Read the model definition and answer for the solid it produces. Units are mm, in the model's axes. A direction names the side the tool comes from. Coordinates: 2 decimals unless noted, no trailing zeros. Order: outer loops, then holes, each group sorted by start corner. A loop starts at its lowest first (then second) coordinate and runs counter-clockwise, first axis right, second up. Notation, with made-up numbers: M 3,-22.75 L 30,-22.75 A22 ccw 30,14.25 Z; hole C 28.5,3.5 d2. An arc over 180 degrees is marked long. Put each result on its own line as item: value.
from build123d import *

# Parameters (mm, degrees)
CYLINDER001_R      = 10.5
CYLINDER001_DEPTH  = 25
CYLINDER_R         = 26
CYLINDER_DEPTH     = 25
CYLINDER002_R      = 30
CYLINDER002_DEPTH  = 5
SKETCH_R           = 6
POCKET_DEPTH       = 40
POLARPATTERN_COUNT = 8


with BuildPart() as cylinder001:
    # Cylinder001 → Cylinder001 (new body)
    with BuildSketch(Plane.XY):
        Circle(CYLINDER001_R)
    extrude(amount=CYLINDER001_DEPTH)


with BuildPart() as cylinder:
    # Cylinder → Cylinder (new body)
    with BuildSketch(Plane.XY):
        Circle(CYLINDER_R)
    extrude(amount=CYLINDER_DEPTH)


with BuildPart() as polarpattern:
    # Cylinder002 → Cylinder002 (new body)
    with BuildSketch(Plane.XY):
        Circle(CYLINDER002_R)
    extrude(amount=CYLINDER002_DEPTH)

    # Fusion: union Cylinder
    add(cylinder.part)

    # Cut: cut Cylinder001
    add(cylinder001.part, mode=Mode.SUBTRACT)

    # Sketch → Pocket (cut)
    with BuildSketch(Plane.XY.offset(25)):
        with Locations((0, 18.25)):
            Circle(SKETCH_R)
    pocket = extrude(amount=-POCKET_DEPTH, mode=Mode.SUBTRACT)

    # PolarPattern: Pocket ×8 about axis
    polarpattern_axis = Axis((0, 0, 25), (0, 0, 1))
    for i in range(1, POLARPATTERN_COUNT):
        add(pocket.rotate(polarpattern_axis, i * 360 / POLARPATTERN_COUNT), mode=Mode.SUBTRACT)


solid = polarpattern.part
Q1. Find section A-A on y = 0. Write down the section's boundary in (x, z), plus the area to 3 significant figures.
Answers below:
outline: M -30,0 L -24.25,0 L -24.25,25 L -26,25 L -26,5 L -30,5 Z; M -12.25,0 L -10.5,0 L -10.5,25 L -12.25,25 Z; M 10.5,0 L 12.25,0 L 12.25,25 L 10.5,25 Z; M 24.25,0 L 30,0 L 30,5 L 26,5 L 26,25 L 24.25,25 Z
area: 215 mm^2
Q2. A tool of negligible diameter and unlimited length cuts with its end or side. For faces 4 (the face through (-9, 25, 5)), 5 (the face through (-29.97, 1.32, 2.46)), from which of +Z, -Z, +X, -X, +Y, -Y can it reach the whole face along a straight path? Write none if from no direction.
Answers below:
face 4: +Z
face 5: +Z, -Z
Q3. Consider line 1 along Y through (x, z) = (0, 19.75); line 2 along Y through (x, z) = (2, 2.25); line 3 along Y through (x, z) = (-11.5, 2.5). Determine where each line is inside the solid, lowest interval first.
Answers below:
line 1: y = -26 to -24.25, -12.25 to -10.5, 10.5 to 12.25, 24.25 to 26
line 2: y = -29.93 to -23.91, -12.59 to -10.31, 10.31 to 12.59, 23.91 to 29.93
line 3: y = -27.71 to -18.74, -7.07 to 7.07, 18.74 to 27.71
Q4. Find section C-C on x = 22. Write down the section's boundary in (y, z), plus the area to 3 significant figures.
Answers below:
outline: M -20.4,0 L -4.68,0 L -4.68,25 L -13.86,25 L -13.86,5 L -20.4,5 Z; M 4.68,0 L 20.4,0 L 20.4,5 L 13.86,5 L 13.86,25 L 4.68,25 Z
area: 524 mm^2
Q5. Find section D-D on z = 3.5. Give the number of separate pieces and of enclosed holes in the cut face, plus the area to 3 significant figures.
Answers below:
separate pieces: 1
enclosed holes: 9
area: 1,580 mm^2
Q6. For a pull along X with two mould halves and no side action, classify faces 1 (the face through (-15.95, 5.54, 12.68)), 2 (the face through (11, 0, 25)), 3 (the face through (-20.633, -15.821, 14.86)) as +X half, -X half, draft (parallel to the pull), parting line (faces both ways), or undercut.
Answers below:
face 1: undercut
face 2: draft
face 3: parting line
Q7. Given pin 1 (6 mm diameter, centred on y = 2.5, z = 17.5, fed in from +X); pin 2 (14 mm diameter, centred on x = -18.25, y = 0, fed in from -Z); pin 3 (2 mm diameter, centred on y = 13.5, z = 3, fed in from -X); pin 4 (3 mm diameter, centred on x = 20, z = 4, fed in from -Y), each flat-ended and moving along its own axis, determine where each tip first touches the part or whether it passes through.
Answers below:
pin 1: stops at x = 26
pin 2: stops at z = 0
pin 3: stops at x = -27.27
pin 4: stops at y = -23.62
